The drawing under review shows one solid part. Ordinate dimensions are in mm from its lowest x, y, z. A direction names the side the tool comes from. Coordinates: 2 decimals unless noted, no trailing zeros. Order: outer loops, then holes, each group sorted by start corner. A loop starts at its lowest first (then second) coordinate and runs counter-clockwise, first axis right, second up.
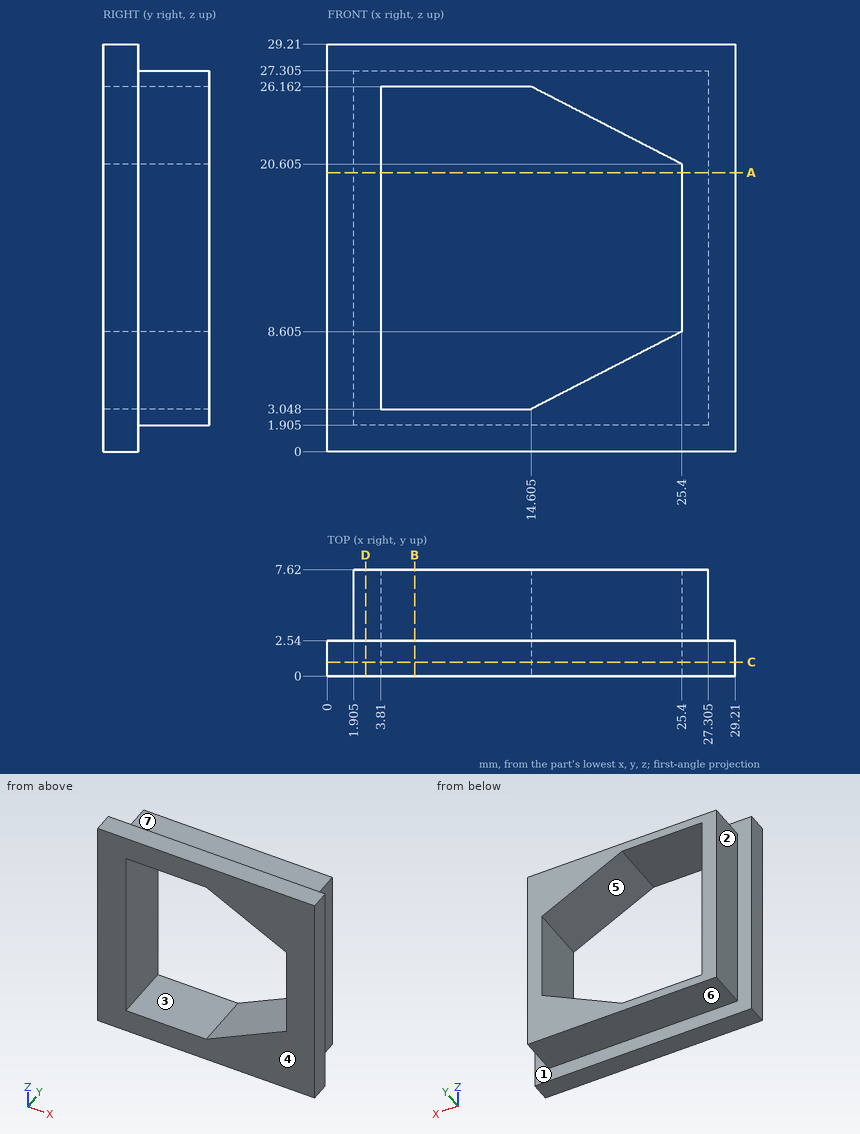
1. Take a section at B-B, the plane x = 6.25. Give the boundary of the cut face in (y, z) (3 decimals), plus the area to 3 significant figures.
Answer below:
outline: (0, 0) - (2.54, 0) - (2.54, 1.905) - (7.62, 1.905) - (7.62, 3.048) - (0, 3.048) - close; (0, 26.162) - (7.62, 26.162) - (7.62, 27.305) - (2.54, 27.305) - (2.54, 29.21) - (0, 29.21) - close
area: 27.1 mm2
2. To check wall thickness, follow L1, parallel to X at y = 7.25, z = 10 (3 decimals); L2, parallel to Z at x = 11, y = 5.5 (3 decimals); L3, parallel to X at y = 1.5, z = 10. State the ranges of each line that lie inside material, in increasing order.
Answer below:
L1: x = 1.905 to 3.81, 25.4 to 27.305
L2: z = 1.905 to 3.048, 26.162 to 27.305
L3: x = 0 to 3.81, 25.4 to 29.21
3. Take a section at A-A, the plane z = 20. Give the boundary of the cut face in (x, y) (3 decimals).
Answer below:
outline: (0, 0) - (3.81, 0) - (3.81, 7.62) - (1.905, 7.62) - (1.905, 2.54) - (0, 2.54) - close; (25.4, 0) - (29.21, 0) - (29.21, 2.54) - (27.305, 2.54) - (27.305, 7.62) - (25.4, 7.62) - close
4. Take a section at D-D, the plane x = 2.75. Give the boundary of the cut face in (y, z) (3 decimals), plus the area to 3 significant figures.
Answer below:
outline: (0, 0) - (2.54, 0) - (2.54, 1.905) - (7.62, 1.905) - (7.62, 27.305) - (2.54, 27.305) - (2.54, 29.21) - (0, 29.21) - close
area: 203 mm2
5. The part is to be moulded in two halves that separate along X. For the marked faces 1, 2 and 3, say which applies: +X half, -X half, draft (parallel to the pull), parting line (faces both ways), or undercut.
Answer below:
face 1: draft
face 2: -X half
face 3: undercut
6. Take a section at C-C, the plane y = 1. Give the boundary of the cut face in (x, z) (3 decimals), plus the area to 3 significant figures.
Answer below:
outline: (0, 0) - (29.21, 0) - (29.21, 29.21) - (0, 29.21) - close; hole (3.81, 3.048) - (14.605, 3.048) - (25.4, 8.605) - (25.4, 20.605) - (14.605, 26.162) - (3.81, 26.162) - close
area: 414 mm2
7. Clearance check with flat-ended pins moving along their axes: pin 1 Ø1.5 at (y, z) = (5.5, 19.5) entering from -X (3 decimals); pin 2 Ø4 at (x, y) = (10, 5.5) entering from +Z (3 decimals); pin 3 Ø1.5 at (y, z) = (5.5, 8) entering from +X (3 decimals). State where each tip first meets the part, or that it passes through.
Answer below:
pin 1: stops at x = 1.905
pin 2: stops at z = 27.305
pin 3: stops at x = 27.305
8. Machinability: for the marked faces 4, 5, 6 and 7, which of the approach directions +Z, -Z, +X, -X, +Y, -Y give a long, thin tool a straight path to every point of the face, cutting with its end or side? Answer none if there is none.
Answer below:
face 4: +Z, -Z, +X, -X, -Y
face 5: +Y, -Y
face 6: -Z, +X, -X, +Y
face 7: +Z, +X, -X, +Y
